Check sheet for the modelled part. Datum: model origin and axes. Units: mm. A direction names the side the tool comes from. Give positions to 0.01 mm unless a question says otherwise; leave off trailing zeros. Order: outer loops, then holes, each group sorted by start corner. A loop starts at its lowest first (then second) coordinate and runs counter-clockwise, first axis right, second up. Notation, with made-up numbers: M 40,8.5 L 79,8.5 A25 cw 79,28.5 Z; hole C 62.25,54.5 d11. An arc over 180 degrees is marked long. Answer in a Markdown table with one row per item. Add a question column.
from build123d import *

# Parameters (mm, degrees)
ESBO_O1_W                                    = 100
ESBO_O1_H                                    = 9.525
RESSALTO_EXTRUS_O1_DEPTH                     = 60
RESSALTO_EXTRUS_O2_DEPTH                     = 4.7625
FILETE1_R                                    = 10
ESBO_O3_R                                    = 4
CORTE_EXTRUS_O1_DEPTH                        = 79.68116436
REBAIXO_PARA_PARAFUSO_COM_CABE_A_PAN_2_COUNT = 2
REBAIXO_PARA_PARAFUSO_COM_CABE_A_PAN_2_PITCH = 60


with BuildPart() as part:
    # Esboço1 → Ressalto-extrusão1 (new body)
    with BuildSketch(Plane(origin=(0, 0, 0), x_dir=(1, 0, 0), z_dir=(0, 1, 0))):
        Rectangle(ESBO_O1_W, ESBO_O1_H)
    extrude(amount=RESSALTO_EXTRUS_O1_DEPTH)

    # Esboço2 → Ressalto-extrusão2 (add, symmetric)
    with BuildSketch(Plane.XY):
        Polygon((-29.85, 0), (-10, 0), (-7.75, -4), (-32.1, -4), align=None)
    ressalto_extrus_o2 = extrude(amount=RESSALTO_EXTRUS_O2_DEPTH, both=True)

    # Espelhar1: Ressalto-extrusão2 across plane
    add(ressalto_extrus_o2.mirror(Plane(origin=(0, 0, 0), x_dir=(0, 0, 1), z_dir=(1, 0, 0))))

    # Filete1
    filete1_edges = [part.edges().sort_by_distance(p)[0] for p in [
        (50, 60, 0),
        (-50, 60, 0),
    ]]
    fillet(filete1_edges, radius=FILETE1_R)

    # Esboço3 → Corte-extrusão1 (cut, through all)
    with BuildSketch(Plane.XY.offset(4.7625)):
        with Locations((-30, 15)):
            Circle(ESBO_O3_R)
        with Locations((30, 15)):
            Circle(ESBO_O3_R)
    extrude(amount=-CORTE_EXTRUS_O1_DEPTH, mode=Mode.SUBTRACT)

    # Esboço9 → Rebaixo para parafuso com cabeça panela de M82 (revolve, cut)
    with BuildSketch(Plane(origin=(30, 15, -4.7625), x_dir=(0, 1, 0), z_dir=(1, 0, 0))):
        Polygon((0, 0), (0, 22.5736146), (4.2, 20.05), (4.2, 6), (9, 6), (9, 0.025), (9.025, 0), align=None)
    rebaixo_para_parafuso_com_cabe_a_panela = revolve(axis=Axis((30, 15, -11.1125), (0, 0, 1)), mode=Mode.SUBTRACT)

    # Rebaixo para parafuso com cabe_a pan 2: Rebaixo para parafuso com cabeça panela de M82 ×2
    with Locations(*[(-i * REBAIXO_PARA_PARAFUSO_COM_CABE_A_PAN_2_PITCH, 0, 0) for i in range(1, REBAIXO_PARA_PARAFUSO_COM_CABE_A_PAN_2_COUNT)]):
        add(rebaixo_para_parafuso_com_cabe_a_panela, mode=Mode.SUBTRACT)


solid = part.part
Q1. Cross-section at A-A (z = 3.25). Record the boundary of the cut face in (x, y).
Q2. Tool access check on faces 5 (the flat face through (-30.99, -2.03, 0.07)), 6 (the cylindrical face through (-37.59, 19.84, -1.79)), 7 (the flat face through (-1, 28, 4.762)), 8 (the flat face through (0, 0, 0)). Record the directions out of +Z, -Z, +X, -X, +Y, -Y that give a thin tool (end or side, any length) a straight path to the whole face; none if there is none.
Q3. Thickness scan on probe 1 along X at (y, z) = (15, 3.85); probe 2 along X at (y, z) = (15, 0.05); probe 3 along Y at (x, z) = (-30, -2.3). Record the ranges inside material, lowest first.
Q4. Draft check along Y on faces 1 (the flat face through (30.99, -2.03, 0.07)), 2 (the flat face through (-1, 28, -4.762)), 3 (the cylindrical face through (-34.164, 14.453, 2.975)), 4 (the flat face through (-20, -4, 0)). Enter one of: pulls with the +Y half, pulls with the -Y half, needs draft (parallel to the pull), parting line crosses it, or undercut.
Q5. Cross-section at B-B (y = 15). State how many separate pieces and enclosed holes the cut face has, and give its area (3 significant figures).
Q6. Go/stop test with flat-tipped pins: pin 1 (3 mm diameter, centred on x = -42.5, z = -1.5, fed in from -Y); pin 2 (9 mm diameter, centred on x = -29, y = 11, fed in from -Z); pin 3 (7.5 mm diameter, centred on x = 30, y = 15, fed in from -Z). Record where each tip stops, or that it passes through.
Q7. Cross-section at C-C (x = -6.5). Record the boundary of the cut face in (y, z), and give its area (4 significant figures).
Values follow:
| question | item | result |
|---|---|---|
| 1 | outline | M -50,0 L -29.85,0 L -32.1,-4 L -7.75,-4 L -10,0 L 10,0 L 7.75,-4 L 32.1,-4 L 29.85,0 L 50,0 L 50,50 A10 ccw 40,60 L -40,60 A10 ccw -50,50 Z; hole C -30,15 d8.4; hole C 30,15 d8.4 |
| 2 | face 5 | +Z, -Z, -X |
| 2 | face 6 | -Z |
| 2 | face 7 | +Z, +X, -X, +Y, -Y |
| 2 | face 8 | +Z, -Z |
| 3 | probe 1 | -50 to -34.2, -25.8 to 25.8, 34.2 to 50 |
| 3 | probe 2 | -50 to -39, -21 to 21, 39 to 50 |
| 3 | probe 3 | -4 to -0.27, 0 to 6, 24 to 60 |
| 4 | face 1 | undercut |
| 4 | face 2 | needs draft |
| 4 | face 3 | undercut |
| 4 | face 4 | pulls with the -Y half |
| 5 | separate pieces | 3 |
| 5 | enclosed holes | 0 |
| 5 | area | 677 mm² |
| 6 | pin 1 | y = 0 |
| 6 | pin 2 | z = 1.24 |
| 6 | pin 3 | through |
| 7 | outline | M 0,-4.76 L 60,-4.76 L 60,4.76 L 0,4.76 Z |
| 7 | area | 571.5 mm² |
